from build123d import *

# Parameters (mm, degrees)
F0_W     = 20
F0_H     = 60
F0_R     = 1.75
F1_DEPTH = 2
F2_W     = 20
F2_H     = 10
F2_R     = 1.75
F3_DEPTH = 6
F5_DEPTH = 2.5


with BuildPart() as f1:
    # F0 (on Top) → F1 (new body)
    with BuildSketch(Plane.XY):
        Rectangle(F0_W, F0_H)
        with Locations((0, -25)):
            Circle(F0_R, mode=Mode.SUBTRACT)
        with Locations((0, 25)):
            Circle(F0_R, mode=Mode.SUBTRACT)
    extrude(amount=F1_DEPTH)

    # F2 (on face) → F3 (join)
    with BuildSketch(Plane.XY.offset(2)):
        with Locations((0, 25)):
            Rectangle(F2_W, F2_H)
        with Locations((0, 25)):
            Circle(F2_R, mode=Mode.SUBTRACT)
        with Locations((0, -25)):
            Rectangle(F2_W, F2_H)
        with Locations((0, -25)):
            Circle(F2_R, mode=Mode.SUBTRACT)
    extrude(amount=F3_DEPTH)

    # F4 (on face) → F5 (cut)
    with BuildSketch(Plane.XY):
        Polygon((1.5877132403, -22.25), (-1.5877132403, -22.25), (-3.1754264805, -25), (-1.5877132403, -27.75), (1.5877132403, -27.75), (3.1754264805, -25), align=None)
        Polygon((1.5877132403, 27.75), (-1.5877132403, 27.75), (-3.1754264805, 25), (-1.5877132403, 22.25), (1.5877132403, 22.25), (3.1754264805, 25), align=None)
    extrude(amount=F5_DEPTH, mode=Mode.SUBTRACT)


solid = f1.part
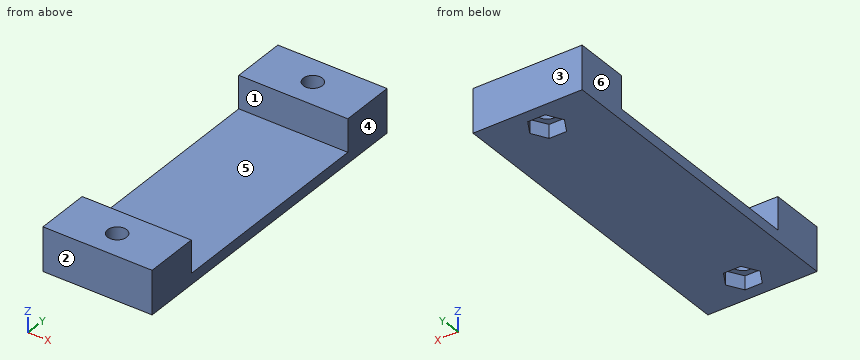
The listing builds one solid part. Answer for the finished solid, in the listing's coordinates (mm). Face numbers are marked on the shaded views. A direction names the side the tool comes from. Round coordinates to 2 decimals unless told otherwise and drop trailing zeros. Write each loop counter-clockwise with the first axis right and the second up, starting at its lowest first coordinate (ties: lowest second). Pieces come first, ordered by that corner, then holes. Notation, with made-up numbers: M 41,47 L 68,47 A18 ccw 68,77 Z; hole C 2.5,11.25 d1. An arc over 180 degrees is marked long. Write each question's results on one line, items separated by ' | '. Start each with the question number.
Item 1: The mould has two halves that part along Y. Classify the marked faces 1, 2, 3 and 4: +Y half, -Y half, draft (parallel to the pull), parting line (faces both ways), or undercut.
Item 2: Which of the six approach directions +Z, -Z, +X, -X, +Y, -Y give full straight-line access (tool end or side, diameter ignored) to the marked faces 5 and 6?
Item 3: Find section D-D on y = 11.5. Write down the section's boundary in (x, z).
Item 4: Find section B-B on x = 0. Write down the section's boundary in (y, z), and give its area (3 significant figures).
Item 5: Given pin 1 Ø3 at (x, y) = (0, 25) entering from +Z; pin 2 Ø4 at (x, y) = (8, 15) entering from +Z; pin 3 Ø6 at (x, y) = (0.5, 26.5) entering from -Z; pin 4 Ø3 at (x, y) = (-0.5, -25) entering from -Z, each flat-ended and moving along its own axis, determine where each tip first touches the part or whether it passes through.
Item 6: Find section A-A on z = 4.25. Write down the section's boundary in (x, y).
Item 7: Straight lines are drawn through the part: probe 1 along Y at (x, z) = (0, 5.7); probe 2 along Y at (x, z) = (8, 6.5); probe 3 along X at (y, z) = (-25, 6.45). For each, find the intervals that lie inside material, in ascending order.
Item 8: Find section C-C on z = 0.75. Write down the section's boundary in (x, y).
Answer block:
1) face 1: undercut | face 2: -Y half | face 3: +Y half | face 4: draft
2) face 5: +Z, +X, -X | face 6: +Z, -Z, -X, +Y, -Y
3) outline: M -10,0 L 10,0 L 10,2 L -10,2 Z
4) outline: M -30,0 L -27.75,0 L -27.75,2.5 L -26.75,2.5 L -26.75,8 L -30,8 Z; M -23.25,2.5 L -22.25,2.5 L -22.25,0 L 22.25,0 L 22.25,2.5 L 23.25,2.5 L 23.25,8 L 20,8 L 20,2 L -20,2 L -20,8 L -23.25,8 Z; M 26.75,2.5 L 27.75,2.5 L 27.75,0 L 30,0 L 30,8 L 26.75,8 Z | area: 174 mm²
5) pin 1: passes through | pin 2: stops at z = 2 | pin 3: stops at z = 0 | pin 4: stops at z = 2.5
6) outline: M -10,-30 L 10,-30 L 10,-20 L -10,-20 Z; M -10,20 L 10,20 L 10,30 L -10,30 Z; hole C 0,-25 d3.5; hole C 0,25 d3.5
7) probe 1: y = -30 to -26.75, -23.25 to -20, 20 to 23.25, 26.75 to 30 | probe 2: y = -30 to -20, 20 to 30 | probe 3: x = -10 to -1.75, 1.75 to 10
8) outline: M -10,-30 L 10,-30 L 10,30 L -10,30 Z; hole M -3.18,-25 L -1.59,-27.75 L 1.59,-27.75 L 3.18,-25 L 1.59,-22.25 L -1.59,-22.25 Z; hole M -3.18,25 L -1.59,22.25 L 1.59,22.25 L 3.18,25 L 1.59,27.75 L -1.59,27.75 Z
